Work out the finished part from the listing and answer in its coordinate system (mm). A direction names the side the tool comes from. Coordinates: 2 decimals unless noted, no trailing zeros. Loops run counter-clockwise (first coordinate to the right, second up) from the corner with the lowest first, then second, coordinate; pieces in that order, holes last. Notation, with made-up numbers: M 22.25,62 L 46.25,62 A9 ccw 46.25,72 Z; hole C 29,-6 d5. An arc over 180 degrees is marked long. Write each question's results on one line, items separated by ' | '.
```python
from build123d import *

# Parameters (mm, degrees)
EXTRUDE_1_DEPTH          = 10
SKETCH_2_R               = 5.5
EXTRUDE_2_DEPTH          = 10
CUT_EXTRUDE_1_DEPTH      = 11.5
CUT_EXTRUDE_3_DEPTH      = 23.837874147
CUT_EXTRUDE_3_DEPTH_BACK = 23.837874147
SKETCH_4_R               = 1.5
SKETCH_6_R               = 1.5
CUT_EXTRUDE_4_DEPTH      = 15.736856398


with BuildPart() as part:
    # 草图1 → 凸台-拉伸1 (new body)
    with BuildSketch(Plane(origin=(0, 0, 0), x_dir=(1, 0, 0), z_dir=(0, 1, 0))):
        Polygon((3.602298117, -5.918061192), (6.926340392, 0.160651085), (3.324042275, 6.078712278), (-3.602298117, 5.918061192), (-6.926340392, -0.160651085), (-3.324042275, -6.078712278), align=None)
    extrude(amount=EXTRUDE_1_DEPTH)

    # 草图2 → 凸台-拉伸2 (add)
    with BuildSketch(Plane(origin=(0, 10, 0), x_dir=(1, 0, 0), z_dir=(0, 1, 0))):
        with Locations(Location((0, 0, 0), (0, 0, 270))):
            Circle(SKETCH_2_R)
    extrude(amount=EXTRUDE_2_DEPTH)

    # 草图3 → 切除-拉伸1 (cut)
    with BuildSketch(Plane(origin=(0, 20, 0), x_dir=(1, 0, 0), z_dir=(0, 1, 0))):
        with BuildLine():
            Line((-1.658312395, -2.5), (1.658312395, -2.5))
            ThreePointArc((1.658312395, -2.5), (0, 3), (-1.658312395, -2.5))
        make_face()
    extrude(amount=-CUT_EXTRUDE_1_DEPTH, mode=Mode.SUBTRACT)

    # 草图4 → 切除-拉伸3 (cut, two sides: drawn at the far end of the back side and taken through both)
    with BuildSketch(Plane(origin=(0, 0, 2.5), x_dir=(-1, 0, 0), z_dir=(0, 0, -1)).offset(-CUT_EXTRUDE_3_DEPTH_BACK)):
        with Locations((0, 17.5)):
            Circle(SKETCH_4_R)
    extrude(amount=CUT_EXTRUDE_3_DEPTH + CUT_EXTRUDE_3_DEPTH_BACK, mode=Mode.SUBTRACT)

    # 草图6 → 切除-拉伸4 (cut, through all)
    with BuildSketch(Plane(origin=(0, 8.5, 0), x_dir=(1, 0, 0), z_dir=(0, 1, 0))):
        with Locations(Location((0, 0, 0), (0, 0, 270))):
            Circle(SKETCH_6_R)
    extrude(amount=-CUT_EXTRUDE_4_DEPTH, mode=Mode.SUBTRACT)


solid = part.part
```
1) Which of the six approach directions +Z, -Z, +X, -X, +Y, -Y give full straight-line access (tool end or side, diameter ignored) to faces 1 (the face through (-2.11, 14.93, 5.08)), 2 (the face through (-2.4, 20, 2.4))?
Check result:
face 1: +Y | face 2: +Z, -Z, +X, -X, +Y
2) Given pin 1 Ø3.5 at (x, y) = (0, 17.5) entering from +Z; pin 2 Ø2.5 at (x, y) = (0.5, 13.5) entering from -Z; pin 3 Ø1.8 at (x, y) = (0, 17.5) entering from -Z; pin 4 Ø2 at (x, z) = (2, 3) entering from -Y, each flat-ended and moving along its own axis, determine where each tip first touches the part or whether it passes through.
Check result:
pin 1: z = 5.5 | pin 2: z = -5.5 | pin 3: through | pin 4: y = 0
3) Straight lines are drawn through the part: probe 1 along Y at (x, z) = (0, 4.35); probe 2 along X at (y, z) = (13.5, 0); probe 3 along Z at (x, y) = (0, 13.5). For each, find the intervals that lie inside material, in ascending order. Write a range as [from, to].
Check result:
probe 1: [0, 16], [19, 20] | probe 2: [-5.5, -3], [3, 5.5] | probe 3: [-5.5, -3], [2.5, 5.5]
4) Find section C-C, the plane y = 17.5. Give the vertices of the cut face in (x, z), and give its area (3 significant figures).
Check result:
outline: M -1.66,2.5 L -1.5,2.5 L -1.5,5.29 A5.5 ccw -1.5,-5.29 L -1.5,-2.6 A3 cw Z; M 1.5,-5.29 A5.5 ccw 1.5,5.29 L 1.5,2.5 L 1.66,2.5 A3 cw 1.5,-2.6 Z | area: 51.4 mm^2
5) For a pull along Z with two mould halves and no side action, classify faces 3 (the face through (-5.24, 4.93, -2.92)), 4 (the face through (0, 8.5, -2)), 5 (the face through (-5.15, 4.93, 3.08)) as released by +Z, released by -Z, zero draft, split by the parting line, or undercut.
Check result:
face 3: released by -Z | face 4: undercut | face 5: released by +Z
6) Find section B-B, the plane x = -1. Give the vertices of the cut face in (y, z).
Check result:
outline: M 0,-5.98 L 10,-5.98 L 10,-5.41 L 16.38,-5.41 L 16.38,-2.83 L 8.5,-2.83 L 8.5,-1.12 L 0,-1.12 Z; M 0,1.12 L 8.5,1.12 L 8.5,2.5 L 16.38,2.5 L 16.38,5.41 L 10,5.41 L 10,6.02 L 0,6.02 Z; M 18.62,-5.41 L 20,-5.41 L 20,-2.83 L 18.62,-2.83 Z; M 18.62,2.5 L 20,2.5 L 20,5.41 L 18.62,5.41 Z
7) Find section A-A, the plane y = 9.75. Give the vertices of the cut face in (x, z), and give its area (3 significant figures).
Check result:
outline: M -6.93,0.16 L -3.6,-5.92 L 3.32,-6.08 L 6.93,-0.16 L 3.6,5.92 L -3.32,6.08 Z; hole M -1.66,2.5 A3 ccw long 1.66,2.5 Z | area: 97.6 mm^2
8) Find section D-D, the plane z = -4.75. Give the vertices of the cut face in (x, y).
Check result:
outline: M -4.24,0 L 4.13,0 L 4.13,10 L 2.77,10 L 2.77,20 L -2.77,20 L -2.77,10 L -4.24,10 Z; hole C 0,17.5 d3
